The model under review builds one solid part; all positions refer to its coordinate system, in mm. Coordinates: 2 decimals unless noted, no trailing zeros. Loops run counter-clockwise (first coordinate to the right, second up) from the corner with the lowest first, then second, coordinate; pieces in that order, holes last. Notation, with made-up numbers: (45, 2) -> (84, 2) arc R21 ccw to (84, 28) -> close; hole circle Ø11 at (0.5, 22.5). An arc over 180 degrees is marked (long way). One line per question, with ' | ' between items. Start each with the question number.
from build123d import *

# Parameters (mm, degrees)
SKETCH1_R           = 3.4289
SKETCH1_R_2         = 1.7144
SKETCH1_R_3         = 2.2226
SKETCH1_W           = 9.398
SKETCH1_H           = 11.0235
SKETCH1_W_2         = 5.0037
SKETCH1_H_2         = 2.4891
BOSS_EXTRUDE1_DEPTH = 2.54
CHAMFER1_SIZE       = 1.27


with BuildPart() as part:
    # Sketch1 → Boss-Extrude1 (new body)
    with BuildSketch(Plane.XY):
        with BuildLine():
            Line((6.434, 7.2517), (-46.4644, 7.2517))
            add(Edge.make_bspline(
                [(-46.4644, 7.2517), (-48.9654, 7.2501), (-51.3771, 6.2567), (-53.1462, 4.4876)],
                knots=[0.3, 0.3, 0.3, 0.3, 0.4, 0.4, 0.4, 0.4], degree=3))
            add(Edge.make_bspline(
                [(-53.1462, 4.4876), (-54.9139, 2.7201), (-55.907, 0.3228), (-55.9054, -2.1769)],
                knots=[0.4, 0.4, 0.4, 0.4, 0.5, 0.5, 0.5, 0.5], degree=3))
            add(Edge.make_bspline(
                [(-55.9054, -2.1769), (-55.9039, -4.7242), (-54.9188, -7.4291), (-53.137, -9.2518)],
                knots=[0.5, 0.5, 0.5, 0.5, 0.6, 0.6, 0.6, 0.6], degree=3))
            add(Edge.make_bspline(
                [(-53.137, -9.2518), (-51.3786, -11.0507), (-48.9824, -12.0793), (-46.4644, -12.0777)],
                knots=[0.6, 0.6, 0.6, 0.6, 0.7, 0.7, 0.7, 0.7], degree=3))
            Line((-46.4644, -12.0777), (6.434, -12.0777))
            add(Edge.make_bspline(
                [(6.434, -12.0777), (8.9516, -12.0761), (11.3581, -11.0449), (13.1151, -9.2429)],
                knots=[0.8, 0.8, 0.8, 0.8, 0.9, 0.9, 0.9, 0.9], degree=3))
            add(Edge.make_bspline(
                [(13.1151, -9.2429), (14.8954, -7.4173), (15.8766, -4.7239), (15.875, -2.1771)],
                knots=[0.9, 0.9, 0.9, 0.9, 1, 1, 1, 1], degree=3))
            add(Edge.make_bspline(
                [(15.875, -2.1771), (15.8735, 0.3223), (14.8775, 2.7305), (13.1074, 4.496)],
                knots=[0, 0, 0, 0, 0.1, 0.1, 0.1, 0.1], degree=3))
            add(Edge.make_bspline(
                [(13.1074, 4.496), (11.3364, 6.2625), (8.9354, 7.2533), (6.434, 7.2517)],
                knots=[0.1, 0.1, 0.1, 0.1, 0.2, 0.2, 0.2, 0.2], degree=3))
        make_face()
        with Locations((2.35, 0.25)):
            Circle(SKETCH1_R, mode=Mode.SUBTRACT)
        with Locations((12.2554, -2.1716)):
            Circle(SKETCH1_R_2, mode=Mode.SUBTRACT)
        with Locations((-43.3701, -3.5091)):
            Circle(SKETCH1_R_3, mode=Mode.SUBTRACT)
        with Locations((-52.2859, -2.1716)):
            Circle(SKETCH1_R_2, mode=Mode.SUBTRACT)
        with Locations((-30.2191, -4.88075)):
            Rectangle(SKETCH1_W, SKETCH1_H, mode=Mode.SUBTRACT)
        Polygon((-15.3715, -0.5328), (-14.6095, 0.2292), (-8.4119, 0.2292), (-7.6499, -0.5328), (-7.6499, -2.4124), (-15.3715, -2.4124), align=None, mode=Mode.SUBTRACT)
        with Locations((-21.27195, -2.26465)):
            Rectangle(SKETCH1_W_2, SKETCH1_H_2, mode=Mode.SUBTRACT)
    extrude(amount=BOSS_EXTRUDE1_DEPTH)

    # Chamfer1
    chamfer1_edges = [part.edges().sort_by_distance(p)[0] for p in [
        (10.541, -2.1716, 2.54),
        (-54.0003, -2.1716, 2.54),
    ]]
    chamfer(chamfer1_edges, length=CHAMFER1_SIZE)


solid = part.part
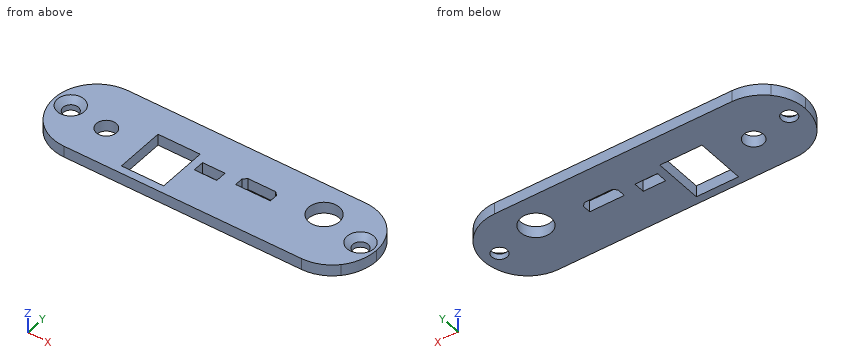
1) Insertion check: pin 1 Ø0.8 at (y, z) = (-6.5, 1.5) entering from +X. The pin has a flat end and moves straight along its axis. Give the tip position at first contact, or say it passes through.
2) Wall thickness on L1, parallel to Y at x = -14, z = 2; L2, parallel to Y at x = -28, z = 1.65; L3, parallel to X at y = -3.25, z = 0.6: over which ranges is each line inside the solid? List them lowest first.
3) Consider section A-A, the plane x = 2.35. Write out the cut boundary in (y, z).
4) Consider section B-B, the plane z = 0.4. Give the number of separate pieces and of enclosed holes in the cut face, plus the area to 3 significant figures.
Filled sheet:
1) pin 1: x = 15.12
2) L1: -12.08 to -2.41, 0.23 to 7.25 | L2: -12.08 to -10.39, 0.63 to 7.25 | L3: -55.85 to -53.62, -50.95 to -45.58, -41.16 to -34.92, -25.52 to -23.77, -18.77 to 10.92, 13.59 to 15.82
3) outline: (-12.08, 0) -> (-3.18, 0) -> (-3.18, 2.54) -> (-12.08, 2.54) -> close; (3.68, 0) -> (7.25, 0) -> (7.25, 2.54) -> (3.68, 2.54) -> close
4) separate pieces: 1 | enclosed holes: 7 | area: 1,100 mm^2
